Geometry check sheet. Reference: drawing and pictorial views, mm from the part's lowest x, y, z. A direction names the side the tool comes from. Give positions to 0.01 mm unless a question says otherwise; leave off trailing zeros. Order: outer loops, then holes, each group sorted by start corner. A loop starts at its lowest first (then second) coordinate and runs counter-clockwise, first axis right, second up.
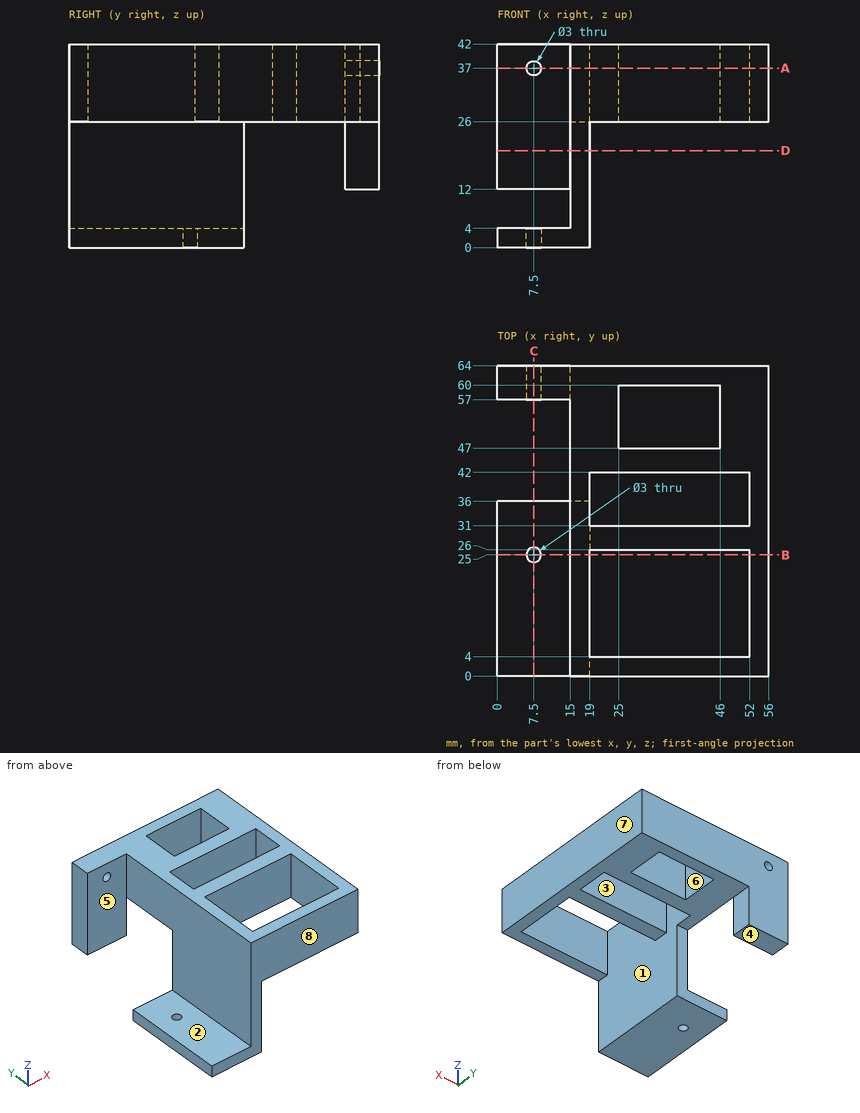
(1) Cross-section at A-A on z = 37. Enter the section's corners in (x, y).
Response values:
outline: (0, 57) - (6, 57) - (6, 64) - (0, 64) - close; (9, 57) - (15, 57) - (15, 0) - (56, 0) - (56, 64) - (9, 64) - close; hole (19, 4) - (52, 4) - (52, 26) - (19, 26) - close; hole (19, 31) - (52, 31) - (52, 42) - (19, 42) - close; hole (25, 47) - (46, 47) - (46, 60) - (25, 60) - close
(2) Release check for a two-part mould opening along X. For the marked faces 6, 7 and 8 record: released by +X, released by -X, zero draft, split by the parting line, or undercut.
Response values:
face 6: undercut
face 7: released by +X
face 8: zero draft
(3) Cross-section at D-D on z = 20. Enter the section's corners in (x, y).
Response values:
outline: (0, 57) - (15, 57) - (15, 64) - (0, 64) - close; (15, 0) - (19, 0) - (19, 36) - (15, 36) - close
(4) Cross-section at C-C on x = 7.5. Enter the section's corners in (y, z).
Response values:
outline: (0, 0) - (23.5, 0) - (23.5, 4) - (0, 4) - close; (26.5, 0) - (36, 0) - (36, 4) - (26.5, 4) - close; (57, 12) - (64, 12) - (64, 35.5) - (57, 35.5) - close; (57, 38.5) - (64, 38.5) - (64, 42) - (57, 42) - close
(5) Gauge pin test, flat ends, axial feed: pin 1 Ø10 at (x, y) = (24.5, 32.5) entering from -Z; pin 2 Ø5.5 at (y, z) = (38, 35) entering from -X; pin 3 Ø12 at (x, y) = (8, 24.5) entering from +Z. Record the tip position at first contact, or that the pin passes through.
Response values:
pin 1: stops at z = 26
pin 2: stops at x = 15
pin 3: stops at z = 4
(6) Set-up check for the marked faces 1, 2, 3, 4 and 5: record each of +Z, -Z, +X, -X, +Y, -Y from which the full face is reachable in a straight line by a thin tool's end or side.
Response values:
face 1: -Z
face 2: +Z, -X, +Y, -Y
face 3: +Z, -Z
face 4: -Z, +X, -X, +Y, -Y
face 5: +Z, -Z, -X, -Y
(7) Cross-section at B-B on y = 25. Enter the section's corners in (x, z), then the cut area to 3 significant figures.
Response values:
outline: (0, 0) - (6, 0) - (6, 4) - (0, 4) - close; (9, 0) - (19, 0) - (19, 42) - (15, 42) - (15, 4) - (9, 4) - close; (52, 26) - (56, 26) - (56, 42) - (52, 42) - close
area: 280 mm2
(8) Material ranges on L1, parallel to Y at x = 28, z = 34; L2, parallel to Y at x = 7.5, z = 1.8; L3, parallel to Y at x = 22.5, z = 37.5, recorded low to high.
Response values:
L1: y = 0 to 4, 26 to 31, 42 to 47, 60 to 64
L2: y = 0 to 23.5, 26.5 to 36
L3: y = 0 to 4, 26 to 31, 42 to 64
